The listing builds one solid part. Answer for the finished solid, in the listing's coordinates (mm). A direction names the side the tool comes from. Coordinates: 2 decimals unless noted, no trailing zeros. Write each loop counter-clockwise with the first axis right and the second up, starting at its lowest first coordinate (ties: lowest second). Pieces come first, ordered by that corner, then holes.
from build123d import *

# Parameters (mm, degrees)
F0_W     = 186.574548
F0_H     = 105.525456
F0_W_2   = 175.490916
F0_H_2   = 89.82364
F1_DEPTH = 101.6
F2_W     = 110.451512
F2_H     = 55.495151
F3_DEPTH = 115.824
F4_R     = 12.681558
F5_DEPTH = 207.264


with BuildPart() as f1:
    # F0 (on Top) → F1 (new body)
    with BuildSketch(Plane.XY):
        Rectangle(F0_W, F0_H)
        Rectangle(F0_W_2, F0_H_2, mode=Mode.SUBTRACT)
    extrude(amount=F1_DEPTH)

    # F2 (on face) → F3 (cut)
    with BuildSketch(Plane.XZ.offset(52.762728)):
        with Locations((0, 75.064696)):
            Rectangle(F2_W, F2_H)
    extrude(amount=-F3_DEPTH, mode=Mode.SUBTRACT)

    # F4 (on face) → F5 (cut)
    with BuildSketch(Plane.YZ.offset(93.287274)):
        with Locations((0, 61.056208)):
            Circle(F4_R)
    extrude(amount=-F5_DEPTH, mode=Mode.SUBTRACT)


solid = f1.part
1. For a pull along Y with two mould halves and no side action, classify faces 4 (the flat face through (-1, 52.763, 39)), 5 (the cylindrical face through (-90.48, -1.65, 73.63)), 6 (the flat face through (-7, -47, 0)) as pulls with the +Y half, pulls with the -Y half, needs draft (parallel to the pull), parting line crosses it, or undercut.
Results found:
face 4: pulls with the +Y half
face 5: undercut
face 6: needs draft
2. A flat-ended cylindrical pin translates along its axis: P1, Ø4, axis at x = 18.5, y = 49, coming from the +Z side. Find the tip coordinate at first contact, or state that the pin passes through.
Results found:
P1: stops at z = 47.32
3. Section A-A on x = 41 is taken. Give the vertices of the cut face in (y, z), then the cut area to 3 significant figures.
Results found:
outline: (-52.76, 0) - (-44.91, 0) - (-44.91, 47.32) - (-52.76, 47.32) - close; (44.91, 0) - (52.76, 0) - (52.76, 47.32) - (44.91, 47.32) - close
area: 743 mm2
4. Section D-D on y = 0 is taken. Give the vertices of the cut face in (x, z).
Results found:
outline: (-93.29, 0) - (-87.75, 0) - (-87.75, 48.37) - (-93.29, 48.37) - close; (-93.29, 73.74) - (-87.75, 73.74) - (-87.75, 101.6) - (-93.29, 101.6) - close; (87.75, 0) - (93.29, 0) - (93.29, 48.37) - (87.75, 48.37) - close; (87.75, 73.74) - (93.29, 73.74) - (93.29, 101.6) - (87.75, 101.6) - close
5. Find the intervals of material crossed by L1, parallel to X at y = -9, z = 76.5; L2, parallel to Y at x = 65, z = 33; L3, parallel to Z at x = -91.3, y = 0, in increasing order.
Results found:
L1: x = -93.29 to -87.75, 87.75 to 93.29
L2: y = -52.76 to -44.91, 44.91 to 52.76
L3: z = 0 to 48.37, 73.74 to 101.6
6. A tool of negligible diameter and unlimited length cuts with its end or side. For faces 1 (the flat face through (-1, 44.912, 39)), 2 (the flat face through (-1, -52.763, 39)), 3 (the flat face through (55.226, -49, 74)), from which of +Z, -Z, +X, -X, +Y, -Y can it reach the whole face along a straight path? Write none if from no direction.
Results found:
face 1: +Z, -Z
face 2: +Z, -Z, +X, -X, -Y
face 3: +Z, +Y, -Y
7. Section B-B on y = 32 is taken. Give the vertices of the cut face in (x, z), then the cut area to 3 significant figures.
Results found:
outline: (-93.29, 0) - (-87.75, 0) - (-87.75, 101.6) - (-93.29, 101.6) - close; (87.75, 0) - (93.29, 0) - (93.29, 101.6) - (87.75, 101.6) - close
area: 1,130 mm2
8. Section C-C on z = 11.5 is taken. Give the vertices of the cut face in (x, y), then the cut area to 3 significant figures.
Results found:
outline: (-93.29, -52.76) - (93.29, -52.76) - (93.29, 52.76) - (-93.29, 52.76) - close; hole (-87.75, -44.91) - (87.75, -44.91) - (87.75, 44.91) - (-87.75, 44.91) - close
area: 3,930 mm2
